Source: CAD feature listing. Evaluate the final solid. Frame: model axes, mm. A direction names the side the tool comes from. Give positions to 0.01 mm unless a question says otherwise; leave off trailing zeros. Loops run counter-clockwise (first coordinate to the right, second up) from the corner with the lowest first, then second, coordinate; pieces in that order, holes last.
```python
from build123d import *

# Parameters (mm, degrees)
SKETCH1_R           = 10
BOSS_EXTRUDE1_DEPTH = 20
SKETCH2_R           = 9
BOSS_EXTRUDE2_DEPTH = 20


with BuildPart() as part:
    # Sketch1 → Boss-Extrude1 (new body)
    with BuildSketch(Plane(origin=(0, 0, 0), x_dir=(0, 0, -1), z_dir=(1, 0, 0))):
        with BuildLine():
            Line((0, 0), (0, -19.63))
            ThreePointArc((0, -19.63), (5.857864376, -33.772135624), (20, -39.63))
            Line((20, -39.63), (118.39773122, -66.572445893))
            ThreePointArc((118.39773122, -66.572445893), (140.164815866, -62.335320368), (150, -42.46))
            Line((150, -42.46), (150, 0))
            Line((150, 0), (0, 0))
        make_face()
        with Locations((20, -19.63)):
            Circle(SKETCH1_R, mode=Mode.SUBTRACT)
        with Locations((125, -42.46)):
            Circle(SKETCH1_R, mode=Mode.SUBTRACT)
    extrude(amount=BOSS_EXTRUDE1_DEPTH)

    # Sketch2 → Boss-Extrude2 (add)
    with BuildSketch(Plane(origin=(0, 0, 0), x_dir=(1, 0, 0), z_dir=(0, 1, 0))):
        with BuildLine():
            Line((0, 150), (-31.593900405, 150))
            ThreePointArc((-31.593900405, 150), (-36.134562655, 149.107762436), (-40, 146.563731056))
            Line((-40, 146.563731056), (-53.965083284, 80.143899292))
            ThreePointArc((-53.965083284, 80.143899292), (-48.911304468, 59.245595573), (-29.5, 50))
            Line((-29.5, 50), (0, 50))
            Line((0, 50), (0, 150))
        make_face()
        with Locations((-29.5, 75)):
            Circle(SKETCH2_R, mode=Mode.SUBTRACT)
    extrude(amount=-BOSS_EXTRUDE2_DEPTH)


solid = part.part
```
(1) Section D-D, the plane x = -18. Return the cut outline in (y, z).
A:
outline: (-20, -150) - (0, -150) - (0, -50) - (-20, -50) - close
(2) Section B-B, the plane z = -76.5. Return the cut outline in (x, y).
A:
outline: (-54.45, -20) - (-38.37, -20) - (-38.37, 0) - (-54.45, 0) - close; (-20.63, -20) - (0, -20) - (0, -55.1) - (20, -55.1) - (20, 0) - (-20.63, 0) - close
(3) Ray query, line 1 along Z through (x, y) = (10, -19); line 2 along Y through (x, z) = (7.5, -125); line 3 along Y through (x, z) = (9, -20). Return the intervals inside material, ascending.
A:
line 1: z = -150 to -29.98, -10.02 to 0
line 2: y = -67.46 to -52.46, -32.46 to 0
line 3: y = -39.63 to -29.63, -9.63 to 0
(4) Section A-A, the plane y = -24. Return the cut outline in (x, z).
A:
outline: (0, -150) - (20, -150) - (20, -28.99) - (0, -28.99) - close; (0, -11.01) - (20, -11.01) - (20, -0.48) - (0, -0.48) - close
(5) First-contact query: pin 1 (23 mm diameter, centred on y = -19.63, z = -20, fed in from -X); pin 2 (2 mm diameter, centred on y = -10.5, z = -94.5, fed in from -X); pin 3 (20.5 mm diameter, centred on x = -29.5, z = -75, fed in from -Y); pin 4 (1.5 mm diameter, centred on x = -14.5, y = -21, fed in from -Z). Flat tips, straight axial feed; report the tip coordinate or a pass-through.
A:
pin 1: stops at x = 0
pin 2: stops at x = -51.16
pin 3: stops at y = -20
pin 4: passes through
(6) Mould query, pull axis Z, two halves, no side actions, for faces 1 (the flat face through (9.86, -52.913, -68.51)), 2 (the flat face through (-46.885, -9.86, -113.819)), 3 (the flat face through (-22, -20, -101)), 4 (the cylindrical face through (-31.451, -9.86, -66.214)). Classes: pulls with the +Z half, pulls with the -Z half, needs draft (parallel to the pull), parting line crosses it, or undercut.
A:
face 1: pulls with the +Z half
face 2: pulls with the -Z half
face 3: needs draft
face 4: undercut
(7) Section C-C, the plane z = -125. Return the cut outline in (x, y), then the cut area to 3 significant figures.
A:
outline: (-44.53, -20) - (0, -20) - (0, -32.46) - (20, -32.46) - (20, 0) - (-44.53, 0) - close; (0, -67.46) - (20, -67.46) - (20, -52.46) - (0, -52.46) - close
area: 1,840 mm2
(8) Reachability of faces 5 (the flat face through (-15, -10, -50)), 6 (the flat face through (-9, 0, -93)) from +Z, -Z, +X, -X, +Y, -Y: full face, straight path, thin tool, end or side. Return the list, or none.
A:
face 5: +Z, -X, +Y, -Y
face 6: +Z, -Z, +X, -X, +Y
